Read the model definition and answer for the solid it produces. Units are mm, in the model's axes. Face numbers are marked on the shaded views. A direction names the side the tool comes from. Coordinates: 2 decimals unless noted, no trailing zeros. Order: outer loops, then holes, each group sorted by start corner. A loop starts at its lowest first (then second) coordinate and runs counter-clockwise, first axis right, second up. Notation, with made-up numbers: (33, 23) - (54, 23) arc R13 ccw to (54, 31) - close; hole circle Ø11 at (19.25, 81). An arc over 180 degrees is marked (long way). Write item = value, one per line.
from build123d import *

# Parameters (mm, degrees)
SKETCH1_W            = 37.8
SKETCH1_H            = 37.8
SKETCH1_W_2          = 33
SKETCH1_H_2          = 33
BOSS_EXTRUDE1_DEPTH  = 9
BOSS_EXTRUDE8_START  = 9
SKETCH8_W            = 37.8
SKETCH8_H            = 37.8
SKETCH8_W_2          = 30.8
SKETCH8_H_2          = 30.8
SKETCH8_W_3          = 26
SKETCH8_H_3          = 26
SKETCH8_W_4          = 22
SKETCH8_H_4          = 22
BOSS_EXTRUDE8_DEPTH  = 2.4
BOSS_EXTRUDE9_START  = 9
SKETCH8_3_W          = 30.8
SKETCH8_3_H          = 30.8
SKETCH8_3_W_2        = 26
SKETCH8_3_H_2        = 26
BOSS_EXTRUDE9_DEPTH  = 5
SKETCH8_4_R          = 1.8288
SKETCH8_4_W          = 37.8
SKETCH8_4_H          = 37.8
BOSS_EXTRUDE10_DEPTH = 9
SKETCH8_5_R          = 1.8288
CUT_EXTRUDE3_DEPTH   = 44.33589736
LPATTERN2_COUNT      = 3
LPATTERN2_PITCH      = 24
LPATTERN2_COUNT_DIR2 = 3
LPATTERN2_PITCH_DIR2 = 24
BOSS_EXTRUDE11_DEPTH = 15.6
CIRPATTERN3_COUNT    = 4


with BuildPart() as part:
    # Sketch1 → Boss-Extrude1 (new, symmetric)
    with BuildSketch(Plane(origin=(0, 0, 0), x_dir=(1, 0, 0), z_dir=(0, 1, 0))):
        Rectangle(SKETCH1_W, SKETCH1_H)
        Rectangle(SKETCH1_W_2, SKETCH1_H_2, mode=Mode.SUBTRACT)
    extrude(amount=BOSS_EXTRUDE1_DEPTH, both=True)

    # Sketch8 → Boss-Extrude8 (add)
    # profile 1 of 3: a face of its own
    with BuildSketch(Plane(origin=(0, 0, 0), x_dir=(1, 0, 0), z_dir=(0, 1, 0)).offset(BOSS_EXTRUDE8_START)):
        Rectangle(SKETCH8_W, SKETCH8_H)
        Rectangle(SKETCH8_W_2, SKETCH8_H_2, mode=Mode.SUBTRACT)
    # profile 2 of 3: a face of its own
    with BuildSketch(Plane(origin=(0, 0, 0), x_dir=(1, 0, 0), z_dir=(0, 1, 0)).offset(BOSS_EXTRUDE8_START)):
        Rectangle(SKETCH8_W_2, SKETCH8_H_2)
        Rectangle(SKETCH8_W_3, SKETCH8_H_3, mode=Mode.SUBTRACT)
    # profile 3 of 3: a face of its own
    with BuildSketch(Plane(origin=(0, 0, 0), x_dir=(1, 0, 0), z_dir=(0, 1, 0)).offset(BOSS_EXTRUDE8_START)):
        Rectangle(SKETCH8_W_3, SKETCH8_H_3)
        Rectangle(SKETCH8_W_4, SKETCH8_H_4, mode=Mode.SUBTRACT)
    extrude(amount=-BOSS_EXTRUDE8_DEPTH)

    # Sketch8<3> → Boss-Extrude9 (add)
    with BuildSketch(Plane(origin=(0, 0, 0), x_dir=(1, 0, 0), z_dir=(0, 1, 0)).offset(BOSS_EXTRUDE9_START)):
        Rectangle(SKETCH8_3_W, SKETCH8_3_H)
        Rectangle(SKETCH8_3_W_2, SKETCH8_3_H_2, mode=Mode.SUBTRACT)
    extrude(amount=BOSS_EXTRUDE9_DEPTH)

    # Sketch8<4> → Boss-Extrude10 (add)
    # profile 1 of 2: a face of its own
    with BuildSketch(Plane(origin=(0, 0, 0), x_dir=(1, 0, 0), z_dir=(0, 1, 0))):
        with BuildLine():
            ThreePointArc((-29, 24), (-27.535533906, 27.535533906), (-24, 29))
            Line((-24, 29), (24, 29))
            ThreePointArc((24, 29), (27.535533906, 27.535533906), (29, 24))
            Line((29, 24), (29, -24))
            ThreePointArc((29, -24), (27.535533906, -27.535533906), (24, -29))
            Line((24, -29), (-24, -29))
            ThreePointArc((-24, -29), (-27.535533906, -27.535533906), (-29, -24))
            Line((-29, -24), (-29, 24))
        make_face()
        with Locations((-24, 24)):
            Circle(SKETCH8_4_R, mode=Mode.SUBTRACT)
        Rectangle(SKETCH8_4_W, SKETCH8_4_H, mode=Mode.SUBTRACT)
    # profile 2 of 2: a face of its own
    with BuildSketch(Plane(origin=(0, 0, 0), x_dir=(1, 0, 0), z_dir=(0, 1, 0))):
        with Locations((-24, 24)):
            Circle(SKETCH8_4_R)
    extrude(amount=-BOSS_EXTRUDE10_DEPTH)

    # Sketch8<5> → Cut-Extrude3 (cut, through all)
    with BuildSketch(Plane(origin=(0, 0, 0), x_dir=(1, 0, 0), z_dir=(0, 1, 0))):
        with Locations(Location((-24, 24, 0), (0, 0, 270))):
            Circle(SKETCH8_5_R)
    cut_extrude3 = extrude(amount=-CUT_EXTRUDE3_DEPTH, mode=Mode.SUBTRACT)

    # LPattern2: Cut-Extrude3 3 × 3
    with Locations(*[(i * LPATTERN2_PITCH, 0, j * LPATTERN2_PITCH_DIR2) for i in range(LPATTERN2_COUNT) for j in range(LPATTERN2_COUNT_DIR2) if (i, j) != (0, 0)]):
        add(cut_extrude3, mode=Mode.SUBTRACT)

    # Sketch10 → Boss-Extrude11 (add)
    with BuildSketch(Plane.XZ.offset(-6.6)):
        with BuildLine():
            Line((-16.5, -11.502376006), (-16.5, -16.5))
            Line((-16.5, -16.5), (-11.502376006, -16.5))
            ThreePointArc((-11.502376006, -16.5), (-12.966146184, -12.966146184), (-16.5, -11.502376006))
        make_face()
    boss_extrude11 = extrude(amount=BOSS_EXTRUDE11_DEPTH)

    # CirPattern3: Boss-Extrude11 ×4 about axis
    cirpattern3_axis = Axis((0, 0, 0), (0, 1, 0))
    for i in range(1, CIRPATTERN3_COUNT):
        add(boss_extrude11.rotate(cirpattern3_axis, i * 360 / CIRPATTERN3_COUNT))


solid = part.part
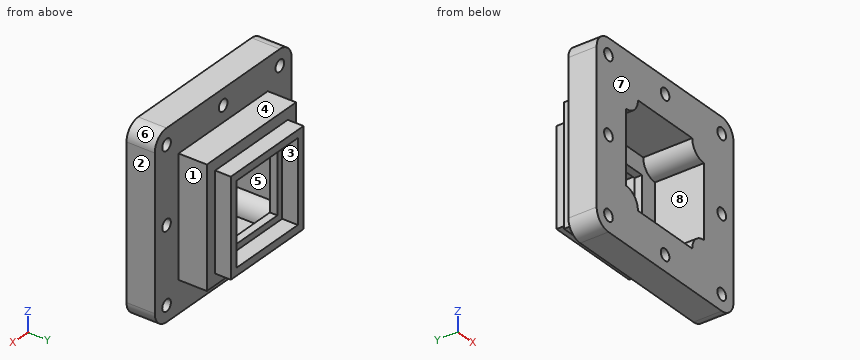
1) Flat-ended cylindrical pins translate along their axes: pin 1 Ø1.5 at (y, z) = (1.5, -20) entering from +X; pin 2 Ø2.5 at (x, y) = (-6.5, 3.5) entering from -Z; pin 3 Ø5 at (y, z) = (6, 18) entering from +X; pin 4 Ø5.5 at (x, y) = (-2.5, 11.5) entering from +Z. Find the tip coordinate at first contact, or state that the pin passes through.
Returned:
pin_1 = through
pin_2 = -18.9
pin_3 = 18.9
pin_4 = 18.9
2) The part is cut by section C-C (z = 18). Determine the outline of the cut face in (x, y).
Returned:
outline = (-29, -9) - (29, -9) - (29, 0) - (18.9, 0) - (18.9, 9) - (-18.9, 9) - (-18.9, 0) - (-29, 0) - close
3) Straight lines are drawn through the part: line 1 along X through (y, z) = (-2, -24); line 2 along X through (y, z) = (-3.5, 0); line 3 along Z through (x, y) = (6, -7.75). For each, find the intervals that lie inside material, in ascending order. Write a range as from..to.
Returned:
line_1 = -29..-25.83, -22.17..-1.83, 1.83..22.17, 25.83..29
line_2 = -29..-25.83, -22.17..-16.5, 16.5..22.17, 25.83..29
line_3 = -29..-16.5, 16.5..29
4) Determine the mould class of the marked faces 6, 7 and 8 for opening direction X: pulls with the +X half, pulls with the -X half, needs draft (parallel to the pull), parting line crosses it, or undercut.
Returned:
face_6 = pulls with the +X half
face_7 = needs draft
face_8 = undercut
5) The part is cut by section B-B (x = 9.5). Determine the outline of the cut face in (y, z), and give its area (3 significant figures).
Returned:
outline = (-9, -29) - (0, -29) - (0, -18.9) - (9, -18.9) - (9, -15.4) - (14, -15.4) - (14, -13) - (9, -13) - (9, -11) - (6.6, -11) - (6.6, -16.5) - (-9, -16.5) - close; (-9, 16.5) - (6.6, 16.5) - (6.6, 11) - (9, 11) - (9, 13) - (14, 13) - (14, 15.4) - (9, 15.4) - (9, 18.9) - (0, 18.9) - (0, 29) - (-9, 29) - close
area = 319 mm^2
6) The part is cut by section A-A (z = 0). Count the separate pieces of the cut face and the enclosed holes in it, and give its area (3 significant figures).
Returned:
separate_pieces = 4
enclosed_holes = 0
area = 253 mm^2
7) For the marked faces 1, 2, 3, 4 and 5, determine the directions among +Z, -Z, +X, -X, +Y, -Y from which every point of the face is accessible in a straight line to the end or side of a thin tool.
Returned:
face_1 = +Z, -Z, +X, +Y
face_2 = +Z, -Z, +X, +Y, -Y
face_3 = +Y
face_4 = +Z, +X, -X, +Y
face_5 = -Y
